Can you work these out from the model? Positions are in its coordinate system, mm. Face numbers are marked on the shaded views. A direction names the side the tool comes from. Round coordinates to 2 decimals unless told otherwise and drop trailing zeros. Loops run counter-clockwise (first coordinate to the right, second up) from the corner with the lowest first, then second, coordinate; pieces in that order, holes last.
(1) I want a section at D-D on x = -1061. Write out the boundary of the cut face in (y, z), plus the area to 3 significant figures.
(2) Will this pin go through, and if not, where does the flat tip stop? pin 1 Ø12 at (x, z) = (-249.5, 596.5) entering from -Y.
(3) I want a section at A-A on x = -762. Write out the boundary of the cut face in (y, z).
(4) I want a section at B-B on y = -66. Write out the boundary of the cut face in (x, z).
(5) I want a section at C-C on z = 778.5. Write out the boundary of the cut face in (x, y), plus the area to 3 significant figures.
(6) Which directions (+Z, -Z, +X, -X, +Y, -Y) give clear straight access to the entire face, cutting with the end or side of a thin tool? Please do the marked faces 5 and 6.
(7) Thinking about a two-plate mould opening in Z: for the marked faces 1, 2, 3 and 4, which applies, released by +Z, released by -Z, zero draft, split by the parting line, or undercut?
(8) If I drill on line 1 along X through (y, z) = (-176, 0); line 2 along Y through (x, z) = (-202, 241.5); line 3 along X through (y, z) = (-156, 165), over which ranges is the centre line in solid material (lowest first)?
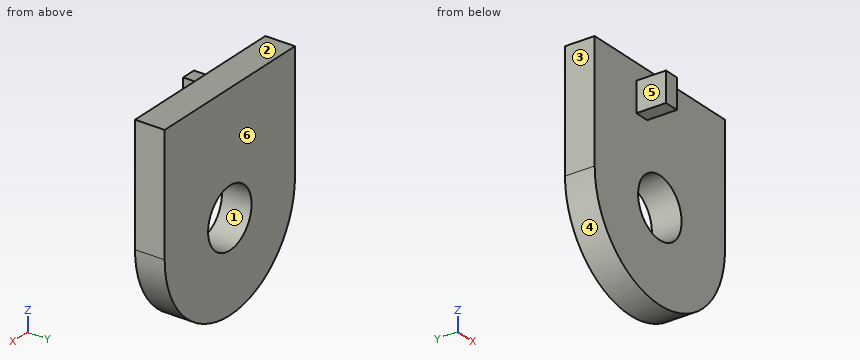
from build123d import *

# Parameters (mm, degrees)
F0_W     = 254
F0_H     = 254
F1_DEPTH = 254
F2_W     = 127
F2_H     = 254
F3_DEPTH = 127
F4_DEPTH = 127


with BuildPart() as f1:
    # F0 (on Front) → F1 (new body)
    with BuildSketch(Plane.XZ):
        Polygon((-254, 1016), (-1524, 1016), (-1524, 254), (-762, 254), (0, 254), (0, 762), (-254, 762), align=None)
        with Locations((-127, 889)):
            Rectangle(F0_W, F0_H)
        with BuildLine():
            Line((-762, 254), (-1524, 254))
            Line((-1524, 254), (-1524, 0))
            ThreePointArc((-1524, 0), (-762, -762), (0, 0))
            Line((0, 0), (0, 254))
            Line((0, 254), (-762, 254))
        make_face()
        with BuildLine():
            ThreePointArc((-508, 0), (-941.6051224214, -179.6051224214), (-762, 254))
            ThreePointArc((-762, 254), (-582.3948775786, 179.6051224214), (-508, 0))
        make_face(mode=Mode.SUBTRACT)
    extrude(amount=F1_DEPTH)

    # F2 (on face) → F3 (join)
    with BuildSketch(Plane.XZ.offset(254)):
        with Locations((-973.7388785046, 748.6669676349)):
            Rectangle(F2_W, F2_H)
    extrude(amount=F3_DEPTH)

    # F4 (add): a face of the model
    f4_faces = [f1.faces().sort_by_distance(p)[0] for p in [
        (-973.7388785046, -381, 748.6669676349),
    ]]
    extrude(f4_faces, amount=F4_DEPTH)


solid = f1.part
Filled sheet:
1. outline: (-254, -700.89) - (0, -700.89) - (0, 1016) - (-254, 1016) - close
1. area: 436,000 mm2
2. pin 1: stops at y = -254
3. outline: (-254, -762) - (0, -762) - (0, -254) - (-254, -254) - close; (-254, 254) - (0, 254) - (0, 1016) - (-254, 1016) - close
4. outline: (-1524, 0) arc R762 ccw to (0, 0) - (0, 1016) - (-1524, 1016) - close; hole circle Ø508 at (-762, 0)
5. outline: (-1524, -254) - (-1037.24, -254) - (-1037.24, -508) - (-910.24, -508) - (-910.24, -254) - (0, -254) - (0, 0) - (-1524, 0) - close
5. area: 419,000 mm2
6. face 5: +Z, -Z, -X, -Y
6. face 6: +Z, -Z, +X, -X, +Y
7. face 1: undercut
7. face 2: released by +Z
7. face 3: zero draft
7. face 4: released by -Z
8. line 1: x = -1524 to -1016, -508 to 0
8. line 2: y = -254 to 0
8. line 3: x = -1524 to -955.11, -568.89 to 0
